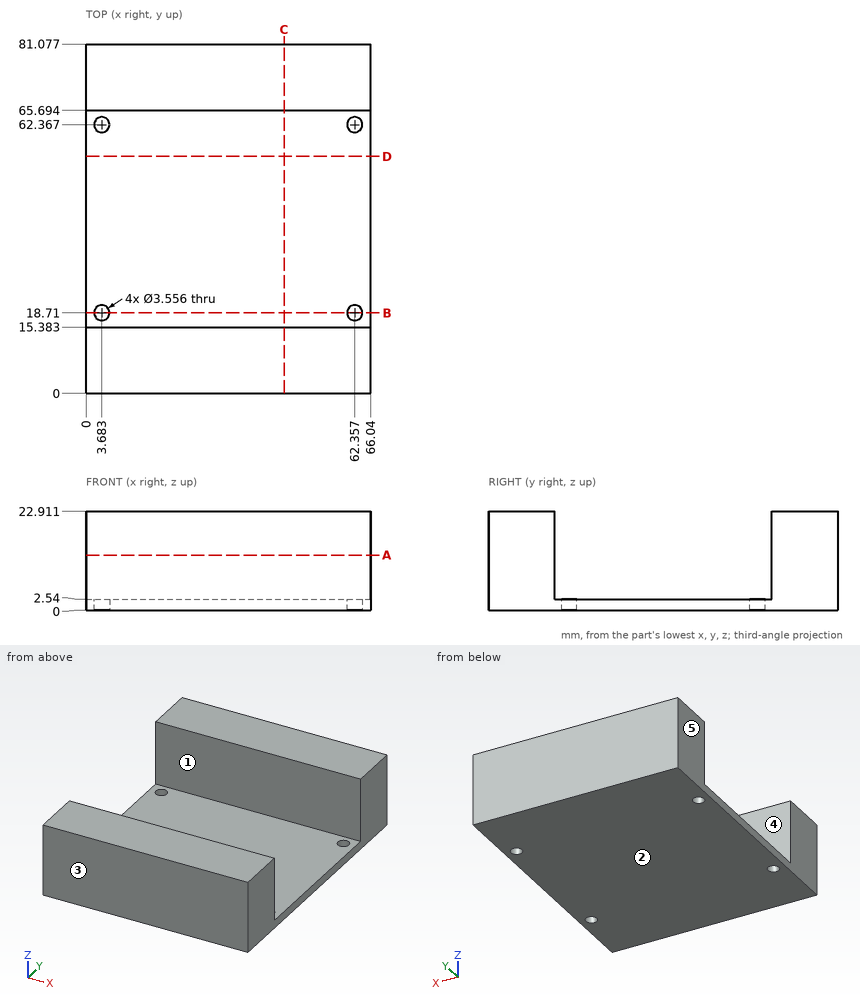
Geometry check sheet. Reference: drawing and pictorial views, mm from the part's lowest x, y, z. A direction names the side the tool comes from. Round coordinates to 2 decimals unless told otherwise and drop trailing zeros. Loops run counter-clockwise (first coordinate to the right, second up) from the corner with the lowest first, then second, coordinate; pieces in that order, holes last.
1. Mould release check, pull along Y, two halves, no side actions. Record for the marked faces 1, 2 and 3: released by +Y, released by -Y, zero draft, split by the parting line, or undercut.
2. Sectioned sample at C-C on x = 46. Record the boundary of the cut face in (y, z).
3. Gauge pin test, flat end, axial feed: pin 1 Ø1.5 at (x, y) = (26, 42.5) entering from +Z. Record the tip position at first contact, or that the pin passes through.
4. Sectioned sample at B-B on y = 18.71. Record the boundary of the cut face in (x, z) (3 decimals), and give its area (3 significant figures).
5. Sectioned sample at D-D on y = 55. Record the boundary of the cut face in (x, z), and give its area (3 significant figures).
6. Set-up check for the marked faces 4 and 5: record each of +Z, -Z, +X, -X, +Y, -Y from which the full face is reachable in a straight line by a thin tool's end or side.
7. Sectioned sample at A-A on z = 12.75. Record the boundary of the cut face in (x, y), and give its area (3 significant figures).
8. Scan lines: probe 1 along Y at (x, z) = (30, 4); probe 2 along Z at (x, y) = (23.5, 19). Record each from-to range of solid material in increasing order.
Recorded:
1. face 1: undercut
1. face 2: zero draft
1. face 3: released by -Y
2. outline: (0, 0) - (81.08, 0) - (81.08, 22.91) - (65.69, 22.91) - (65.69, 2.54) - (15.38, 2.54) - (15.38, 22.91) - (0, 22.91) - close
3. pin 1: stops at z = 2.54
4. outline: (0, 0) - (1.905, 0) - (1.905, 2.54) - (0, 2.54) - close; (5.461, 0) - (60.579, 0) - (60.579, 2.54) - (5.461, 2.54) - close; (64.135, 0) - (66.04, 0) - (66.04, 2.54) - (64.135, 2.54) - close
4. area: 150 mm2
5. outline: (0, 0) - (66.04, 0) - (66.04, 2.54) - (0, 2.54) - close
5. area: 168 mm2
6. face 4: +Z, +X, -X
6. face 5: +Z, -Z, -X, +Y, -Y
7. outline: (0, 0) - (66.04, 0) - (66.04, 15.38) - (0, 15.38) - close; (0, 65.69) - (66.04, 65.69) - (66.04, 81.08) - (0, 81.08) - close
7. area: 2,030 mm2
8. probe 1: y = 0 to 15.38, 65.69 to 81.08
8. probe 2: z = 0 to 2.54
